Print and shaded views of the part. All mm, measured from the part's lowest x, y and z. A direction names the side the tool comes from. Round coordinates to 2 decimals unless told otherwise and drop trailing zeros. Order: outer loops, then holes, each group sorted by start corner. A loop starts at its lowest first (then second) coordinate and runs counter-clockwise, first axis right, second up. Notation, with made-up numbers: (24, 28.25) - (30, 28.25) arc R15 cw to (30, 34.25) - close; hole circle Ø11 at (89, 24). An arc over 180 degrees is marked (long way). Return JSON: item names as keys, results as strings. Group by question number.
Item 1: Tool access for the marked faces 1 and 2: list every direction of +Z, -Z, +X, -X, +Y, -Y with a clear straight run to the whole face (end or side of a thin tool).
Item 2: Probe probe 1 along Y at (x, z) = (15, 3.25); probe 2 along Y at (x, z) = (15, 12.65); probe 3 along Z at (x, y) = (28.5, 19.25). List the from-to ranges inside material, lowest first.
Item 3: Saw through at A-A on x = 15. List the corners of the cut face in (y, z).
Item 4: Saw through at C-C on z = 7.75. List the corners of the cut face in (x, y).
Item 5: Two-plate mould, pull along Y, no slides. Class the marked faces 3, 4 and 5: released by +Y, released by -Y, zero draft, split by the parting line, or undercut.
Item 6: Drop flat-ended pins along their axis: pin 1 (1.5 mm diameter, centred on y = 17, z = 8, fed in from -X); pin 2 (15 mm diameter, centred on x = 15, y = 15, fed in from +Z); pin 3 (6 mm diameter, centred on x = 9, z = 12.5, fed in from -Y); pin 4 (9.5 mm diameter, centred on x = 15, y = 15, fed in from +Z). Give the stop position or say it passes through.
Item 7: Saw through at D-D on z = 12.5. List the corners of the cut face in (x, y).
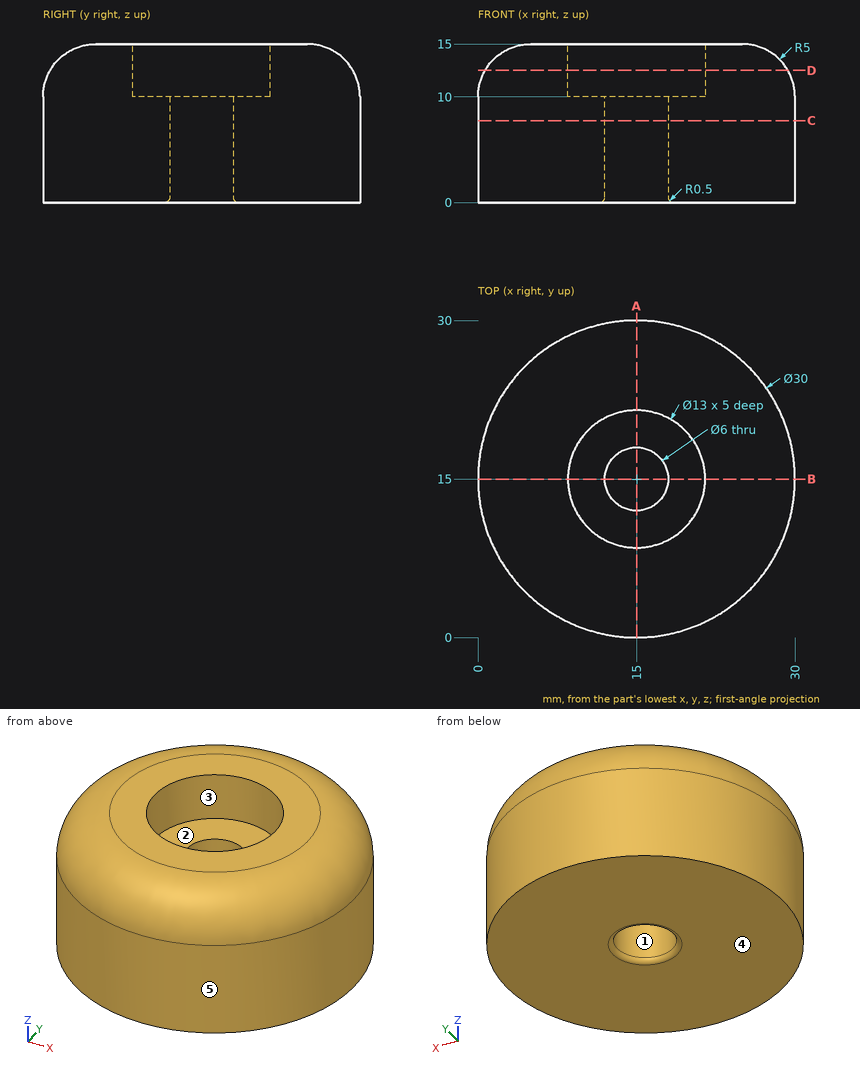
Filled in:
{
 "1": {"face 1": "+Z, -Z", "face 2": "+Z"},
 "2": {"probe 1": "y = 0 to 12, 18 to 30", "probe 2": "y = 0.76 to 8.5, 21.5 to 29.24", "probe 3": "z = 0 to 12.78"},
 "3": {"outline": "(0, 0) - (11.5, 0) arc R0.5 ccw to (12, 0.5) - (12, 10) - (8.5, 10) - (8.5, 15) - (5, 15) arc R5 ccw to (0, 10) - close; (18, 0.5) arc R0.5 ccw to (18.5, 0) - (30, 0) - (30, 10) arc R5 ccw to (25, 15) - (21.5, 15) - (21.5, 10) - (18, 10) - close"},
 "4": {"outline": "circle Ø30 at (15, 15); hole circle Ø6 at (15, 15)"},
 "5": {"face 3": "undercut", "face 4": "zero draft", "face 5": "split by the parting line"},
 "6": {"pin 1": "stops at x = 0.05", "pin 2": "stops at z = 15", "pin 3": "stops at y = 0.49", "pin 4": "stops at z = 10"},
 "7": {"outline": "circle Ø28.66 at (15, 15); hole circle Ø13 at (15, 15)"}
}
